Source: CAD feature listing. Evaluate the final solid. Frame: model axes, mm. A direction names the side the tool comes from. Give positions to 0.01 mm unless a question says otherwise; leave off trailing zeros. Order: outer loops, then holes, each group sorted by start corner. A loop starts at its lowest first (then second) coordinate and runs counter-clockwise, first axis right, second up.
Autodesk Inventor part; units mm, degrees
ref_plane "Work Plane2" through (2.032, 0, 0) normal (0, 1, 0) x (1, 0, 0)
ref_plane "YZ Plane" through (0, 0, 0) normal (1, 0, 0) x (0, 1, 0)
ref_plane "XZ Plane" through (0, 0, 0) normal (0, 1, 0) x (-1, 0, 0)
sketch "Sketch1" plane through (0, 0, 0) normal (0, 0, 1) x (1, 0, 0)
  line L0 (2.6924, 0) -> (9.525, 0)
  line L1 (9.525, 0) -> (9.525, 1.7526)
  line L2 (9.525, 1.7526) -> (2.1082, 1.7526)
  line L3 (0.5596, 3.0988) -> (0, 3.0988)
  line L4 (-1.905, 0) -> (11.43, 0)
  line L5 (0, -0.6198) -> (0, 3.7186)
  line L6 (0, 2.2098) -> (2.0648, 1.1803)
  line L7 (2.0648, 1.1803) -> (2.6924, 0)
  line L8 (2.1082, 1.7526) -> (0.5596, 3.0988)
  line L9 (0, 3.0988) -> (0, 2.2098)
  dimension "d2" = 3.5052
  dimension "d3" = 6.1976
  dimension "d4" = 2.6924
  dimension "d5" = 4.4196
  dimension "d6" = 26.5
  dimension "d7" = 62
  dimension "d13" = 41
  dimension "d14" = 2.1082
  dimension "d15" = 9.525
revolve "Body" add sketch "Sketch1" angle 360 about axis through (2.6924, 0, 0) along (1, 0, 0) contours L7 L6 L5 L3 L8 L2 L1 L0
sketch "Sketch2" plane through (0, 0, 0) normal (-1, 0, 0) x (0, 0, 1)
  line L0 (0, -4.3383) -> (0, 4.3383)
  line L1 (-4.3383, 0) -> (4.3383, 0)
  line L2 (0, 2.2098) -> (0, 0) construction
  line L3 (0, 0) -> (2.2098, 0) construction
  arc A0 (0.7366, 0) -> (0, 0.7366) centre (0, 0) ccw
  line L4 (0, 0) -> (0.7947, 0.7947) construction
  arc A1 (1.1049, 0) -> (0, 1.1049) centre (0, 0) ccw construction
  line L5 (0.3683, 2.1789) -> (0.3131, 1.0596)
  line L6 (2.1789, 0.3683) -> (1.0596, 0.3131)
  arc A2 (0.3131, 1.0596) -> (1.0596, 0.3131) centre (1.0245, 1.0245) ccw
  arc A3 (2.2098, 0) -> (2.1789, 0.3683) centre (0, 0) ccw
  arc A4 (0.3683, 2.1789) -> (0, 2.2098) centre (0, 0) ccw
  arc A5 (2.1789, 0.3683) -> (0.3683, 2.1789) centre (0, 0) ccw
  line L7 (0.3683, -2.1789) -> (0.3131, -1.0596)
  line L8 (2.1789, -0.3683) -> (1.0596, -0.3131)
  arc A6 (1.0596, -0.3131) -> (0.3131, -1.0596) centre (1.0245, -1.0245) ccw
  arc A7 (2.1789, -0.3683) -> (2.2098, 0) centre (0, 0) ccw
  arc A8 (0, -2.2098) -> (0.3683, -2.1789) centre (0, 0) ccw
  arc A9 (0.3683, -2.1789) -> (2.1789, -0.3683) centre (0, 0) ccw
  line L9 (-0.3683, 2.1789) -> (-0.3131, 1.0596)
  line L10 (-2.1789, 0.3683) -> (-1.0596, 0.3131)
  arc A10 (-1.0596, 0.3131) -> (-0.3131, 1.0596) centre (-1.0245, 1.0245) ccw
  arc A11 (-2.1789, 0.3683) -> (-2.2098, 0) centre (0, 0) ccw
  arc A12 (0, 2.2098) -> (-0.3683, 2.1789) centre (0, 0) ccw
  arc A13 (-0.3683, 2.1789) -> (-2.1789, 0.3683) centre (0, 0) ccw
  arc A14 (-2.1789, -0.3683) -> (-0.3683, -2.1789) centre (0, 0) ccw
  arc A15 (-0.3683, -2.1789) -> (0, -2.2098) centre (0, 0) ccw
  arc A16 (-2.2098, 0) -> (-2.1789, -0.3683) centre (0, 0) ccw
  line L11 (-2.1789, -0.3683) -> (-1.0596, -0.3131)
  arc A17 (-0.3131, -1.0596) -> (-1.0596, -0.3131) centre (-1.0245, -1.0245) ccw
  line L12 (-0.3683, -2.1789) -> (-0.3131, -1.0596)
  dimension "d18" = 45
  dimension "d19" = 1.4732
  dimension "d20" = 2.2098
  dimension "d21" = 4.4196
  dimension "d22" = 0.3683
extrude "Slot" add sketch "Sketch2" against normal up to next contours A2 L5 A5 L6 | L9 A10 L10 A13 | L7 A6 L8 A9 | A14 L11 A17 L12
fillet "Fillet1" radius 0.1473 4 edges at (0, 2.2098, 0) (0, 0, 2.2098) (0, -2.2098, 0) (0, 0, -2.2098)
thread "Thread"
chamfer "Chamfer1" distance 0.5953 distance2 0.5953 1 edges at (9.525, -1.7526, 0) measured on face at (9.525, 0.2072, 0.5462)
ref_plane "Work Plane2" through (2.032, 0, 0) normal (0, 1, 0) x (1, 0, 0)
equation "\"d2\" = GD"
equation "\"d3\" = KOD"
equation "\"d4\" = INTI"
equation "\"d5\" = SDM"
equation "\"d13\" = 0.5 * SEWI"
equation "\"d14\" = KOH"
equation "\"d15\" = NLG"
equation "\"d19\" = 0.333333 * SDM"
equation "\"d20\" = 0.5 * SDM"
equation "\"d21\" = SDM"
equation "\"d22\" = 0.5 * SBR"
equation "\"d45\" = INTI"
equation "\"d25\" = 0.2 * SBR"
equation "\"d9\" = GEL"
equation "\"d11\" = -0.5 * SPD + 0.5 * GD"
equation "\"d12\" = GUL"
equation "\"GD\" = NND"
equation "\"NLG\" = 9.525"
equation "\"GEL\" = 5.43243"
equation "\"KOD\" = 6.1976"
equation "\"KOH\" = 2.1082"
equation "\"SDM\" = 4.4196"
equation "\"INTI\" = 2.6924"
equation "\"SBR\" = 0.7366"
equation "\"GUL\" = 0.75 * GAL"
equation "\"SPD\" = 2.31458"
equation "\"SEWI\" = 82deg"
equation "\"d0\" = NLG"
equation "\"d1\" = KOH"
equation "\"d17\" = SDM"
equation "\"TOA\" = 30deg"
equation "\"THREADDIA\" = 3.5052"
equation "\"BDM\" = NND"
equation "\"NND\" = 3.5052"
equation "\"GAL\" = 0.79375"
equation "\"GD1\" = SPD"
properties part number "ANSI B18.6.3 - 6-32 x 3/8, CRFCHMSTII(5)" material "Steel, Mild"
(1) Line query: line 1 along X through (y, z) = (2, 0.5); line 2 along Z through (x, y) = (1.75, 1); line 3 along Z through (x, y) = (8.5, 0). Output: solid intervals per line, ascending.
(2) Pin query (flat end, axial travel): pin 1 Ø1 at (x, z) = (4, -1.5) entering from -Y; pin 2 Ø1 at (y, z) = (-1.5, -0.5) entering from -X. Return the tip coordinate at first contact, or that it passes through.
(3) Section A-A, the plane x = 3. Return loops of the section in (y, z), plus the area to 3 significant figures.
(4) Access query for faces 1 (the cylindrical face through (5.47, 1.67, -0.53)), 2 (the flat face through (0.8, 0.33, 1.4)), 3 (the flat face through (9.525, 0, 0)). Directions: +Z, -Z, +X, -X, +Y, -Y. A direction counts if a zero-diameter tool reaches every point of the face in a straight line with its end or side. Return the directions, or none.
(5) Draft query along Y for faces 4 (the cylindrical face through (0.28, 2.86, 1.19)), 5 (the conical face through (1.06, -1.68, -0.01)), 6 (the flat face through (0.8, 1.4, 0.33)), 7 (the flat face through (0, 1, -1)). Return one class per face: +Y half, -Y half, draft (parallel to the pull), parting line (faces both ways), or undercut.
Checks:
1. line 1: x = 0 to 1.75
1. line 2: z = -1.81 to -0.31, 0.31 to 1.81
1. line 3: z = -1.75 to 1.75
2. pin 1: stops at y = -1.44
2. pin 2: stops at x = 0
3. outline: circle Ø3.51 at (0, 0)
3. area: 9.65 mm2
4. face 1: +X
4. face 2: -X
4. face 3: +Z, -Z, +X, +Y, -Y
5. face 4: parting line
5. face 5: undercut
5. face 6: undercut
5. face 7: draft
